Could you check a few things on this model? Use its own coordinates, in mm. Face numbers are marked on the shaded views. A direction names the side the tool comes from. Coordinates: 2 decimals unless noted, no trailing zeros. Loops run counter-clockwise (first coordinate to the right, second up) from the corner with the lowest first, then second, coordinate; pieces in that order, holes last.
1) Imagine slicing it at B-B on z = 5. Please give me the cut outline in (x, y), plus the area to 3 significant figures.
2) Thinking about a two-plate mould opening in X: for the marked faces 1, 2, 3 and 4, which applies, released by +X, released by -X, zero draft, split by the parting line, or undercut?
3) Imagine slicing it at D-D on x = 33. Please give me the cut outline in (y, z), plus the area to 3 significant figures.
4) For the marked faces 5 and 6, which set-ups out of +Z, -Z, +X, -X, +Y, -Y let a thin tool reach every point of the face, with its end or its side?
5) Imagine slicing it at A-A on y = 2. Please give me the cut outline in (x, z), plus the area to 3 significant figures.
6) Imagine slicing it at C-C on x = -6. Please give me the cut outline in (y, z), plus the area to 3 significant figures.
7) Will these pins go through, and if not, where does the flat tip stop? P1, Ø2, axis at y = 7.76, z = 5, coming from the -X side; P2, Ø4.5, axis at y = 7.76, z = 5, coming from the +X side; P3, Ø1.4, axis at y = 0, z = 5.5, coming from the +X side.
8) If I drill on line 1 along Y through (x, z) = (-13.15, 5); line 2 along X through (y, z) = (5.75, 7.25); line 3 along Y through (x, z) = (10, 7.25), over which ranges is the centre line in solid material (lowest first)?
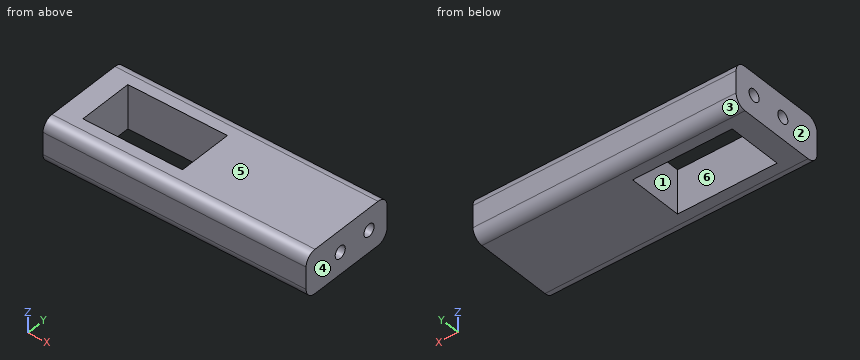
```python
from build123d import *

# Parameters (mm, degrees)
ESBO_O1_W                = 60
ESBO_O1_H                = 22.5
ESBO_O1_W_2              = 22.7
ESBO_O1_H_2              = 12.5
RESSALTO_EXTRUS_O1_DEPTH = 10
ESBO_O3_R                = 1.4
CORTE_EXTRUS_O2_DEPTH    = 20
ESBO_O4_R                = 1.4
CORTE_EXTRUS_O3_DEPTH    = 3
FILETE1_R                = 2.5


with BuildPart() as part:
    # Esboço1 → Ressalto-extrusão1 (new body)
    with BuildSketch(Plane.XY):
        with Locations((14.794474124, 1.507916667)):
            Rectangle(ESBO_O1_W, ESBO_O1_H)
        with Locations((1.144474124, 1.507916667)):
            Rectangle(ESBO_O1_W_2, ESBO_O1_H_2, mode=Mode.SUBTRACT)
    extrude(amount=RESSALTO_EXTRUS_O1_DEPTH)

    # Esboço3 → Corte-extrusão2 (cut)
    with BuildSketch(Plane(origin=(44.794474124, 0, 0), x_dir=(0, 0, -1), z_dir=(1, 0, 0))):
        with Locations((-5, 7.757916667)):
            Circle(ESBO_O3_R)
        with Locations((-5, -0.242083333)):
            Circle(ESBO_O3_R)
    extrude(amount=-CORTE_EXTRUS_O2_DEPTH, mode=Mode.SUBTRACT)

    # Esboço4 → Corte-extrusão3 (cut)
    with BuildSketch(Plane.ZY.offset(15.205525876)):
        with Locations((5, 7.757916667)):
            Circle(ESBO_O4_R)
        with Locations((5, -0.242083333)):
            Circle(ESBO_O4_R)
    extrude(amount=-CORTE_EXTRUS_O3_DEPTH, mode=Mode.SUBTRACT)

    # Filete1
    filete1_edges = [part.edges().sort_by_distance(p)[0] for p in [
        (14.794474124, 12.757916667, 10),
        (14.794474124, 12.757916667, 0),
        (14.794474124, -9.742083333, 0),
        (14.794474124, -9.742083333, 10),
    ]]
    fillet(filete1_edges, radius=FILETE1_R)


solid = part.part
```
Filled in:
1. outline: (-15.21, -9.74) - (44.79, -9.74) - (44.79, -1.64) - (24.79, -1.64) - (24.79, 1.16) - (44.79, 1.16) - (44.79, 6.36) - (24.79, 6.36) - (24.79, 9.16) - (44.79, 9.16) - (44.79, 12.76) - (-15.21, 12.76) - (-15.21, 9.16) - (-12.21, 9.16) - (-12.21, 6.36) - (-15.21, 6.36) - (-15.21, 1.16) - (-12.21, 1.16) - (-12.21, -1.64) - (-15.21, -1.64) - close; hole (-10.21, -4.74) - (12.49, -4.74) - (12.49, 7.76) - (-10.21, 7.76) - close
1. area: 937 mm2
2. face 1: undercut
2. face 2: released by -X
2. face 3: zero draft
2. face 4: released by +X
3. outline: (-9.74, 2.5) arc R2.5 ccw to (-7.24, 0) - (10.26, 0) arc R2.5 ccw to (12.76, 2.5) - (12.76, 7.5) arc R2.5 ccw to (10.26, 10) - (-7.24, 10) arc R2.5 ccw to (-9.74, 7.5) - close; hole circle Ø2.8 at (-0.24, 5); hole circle Ø2.8 at (7.76, 5)
3. area: 207 mm2
4. face 5: +Z, +X, -X, +Y, -Y
4. face 6: +Z, -Z
5. outline: (-15.21, 0) - (-10.21, 0) - (-10.21, 10) - (-15.21, 10) - close; (12.49, 0) - (44.79, 0) - (44.79, 10) - (12.49, 10) - close
5. area: 373 mm2
6. outline: (-9.74, 2.5) arc R2.5 ccw to (-7.24, 0) - (-4.74, 0) - (-4.74, 10) - (-7.24, 10) arc R2.5 ccw to (-9.74, 7.5) - close; (7.76, 0) - (10.26, 0) arc R2.5 ccw to (12.76, 2.5) - (12.76, 7.5) arc R2.5 ccw to (10.26, 10) - (7.76, 10) - close
6. area: 94.6 mm2
7. P1: stops at x = -12.21
7. P2: stops at x = 44.79
7. P3: stops at x = 24.79
8. line 1: y = -9.74 to -1.64, 1.16 to 6.36, 9.16 to 12.76
8. line 2: x = -15.21 to -10.21, 12.49 to 44.79
8. line 3: y = -9.74 to -4.74, 7.76 to 12.76
